Build history of the part. All positions in model axes, mm. A direction names the side the tool comes from. Round coordinates to 2 decimals unless told otherwise and drop trailing zeros. Write each loop counter-clockwise with the first axis right and the second up, starting at its lowest first coordinate (ties: lowest second). Pieces come first, ordered by that corner, then holes. Notation, with made-up numbers: (49.25, 19.5) - (54.25, 19.5) arc R26 cw to (54.25, 35.5) - close; hole circle Ø7 at (51.25, -8). An arc over 180 degrees is marked (long way). Answer as a JSON object with one key per item and string values. Group by question number.
Item 1: Two-plate mould, pull along Y, no slides. Class faces 4 (the flat face through (-1, -11.684, -3)), 5 (the cylindrical face through (4.851, -9.945, -0.888)), 6 (the cylindrical face through (-4.841, -9.117, 0.41)), 7 (the flat face through (-5.207, -10, 0)): +Y half, -Y half, draft (parallel to the pull), parting line (faces both ways), or undercut.
Item 2: Flat gauge pins, fed straight in: pin 1 (1.5 mm diameter, centred on x = 3, z = 0.5, fed in from -Y); pin 2 (5 mm diameter, centred on y = 8.5, z = -4, fed in from -X); pin 3 (1.5 mm diameter, centred on x = -2.5, y = 1.5, fed in from -Z). Where does each tip first touch, or does it go through?
Item 3: Probe line 1 (Y direction, x = -2, z = -4.5); line 2 (Z direction, x = 0, y = 6.5); line 3 (Z direction, x = -2.75, y = 1.25). List the from-to ranges inside material, lowest first. Write a range as from..to.
Item 4: Slice it at B-B, the plane y = 3.5. List the corners of the cut face in (x, z), then the cut area to 3 significant figures.
Item 5: Which spindle directions (+Z, -Z, +X, -X, +Y, -Y) get a long thin tool onto all of the face, cutting with end or side? Do faces 1 (the flat face through (5.207, -10, 0)), 2 (the cylindrical face through (-2.092, 1.002, -5.045)), 3 (the flat face through (-5, 2.032, 0)). Say none if no direction does.
Item 6: Slice it at A-A, the plane y = -6. List the corners of the cut face in (x, z).
from build123d import *

# Parameters (mm, degrees)
SKETCH2_R           = 4.826
BOSS_EXTRUDE1_DEPTH = 15.494
FILLET1_R           = 4.826
SKETCH3_R           = 5.461
BOSS_EXTRUDE2_DEPTH = 2.032
SKETCH4_R           = 4.572
BOSS_EXTRUDE3_DEPTH = 11.684
SKETCH5_R           = 2.921
BOSS_EXTRUDE4_DEPTH = 2.794
BOSS_EXTRUDE4_TAPER = 35
FILLET2_R           = 1.27
FILLET3_R           = 0.508
SKETCH6_R           = 0.889
BOSS_EXTRUDE5_DEPTH = 5.207


with BuildPart() as part:
    # Sketch2 → Boss-Extrude1 (new body)
    with BuildSketch(Plane(origin=(0, 0, 0), x_dir=(1, 0, 0), z_dir=(0, 1, 0))):
        with Locations(Location((0, 0, 0), (0, 0, 270))):  # turned: the seam where the file's is
            Circle(SKETCH2_R)
    extrude(amount=BOSS_EXTRUDE1_DEPTH)

    # Fillet1
    fillet1_edges = [part.edges().sort_by_distance(p)[0] for p in [
        (0, 15.494, -4.826),
    ]]
    fillet(fillet1_edges, radius=FILLET1_R)

    # Sketch3 → Boss-Extrude2 (add)
    with BuildSketch(Plane.XZ):
        with Locations(Location((0, 0, 0), (0, 0, 270))):  # turned: the seam where the file's is
            Circle(SKETCH3_R)
    extrude(amount=-BOSS_EXTRUDE2_DEPTH)

    # Sketch4 → Boss-Extrude3 (add)
    with BuildSketch(Plane.XZ):
        with Locations(Location((0, 0, 0), (0, 0, 90))):  # turned: the seam where the file's is
            Circle(SKETCH4_R)
    extrude(amount=BOSS_EXTRUDE3_DEPTH)

    # Sketch5 → Boss-Extrude4 (add)
    with BuildSketch(Plane.XZ.offset(11.684)):
        Circle(SKETCH5_R)
    extrude(amount=BOSS_EXTRUDE4_DEPTH, taper=BOSS_EXTRUDE4_TAPER)

    # Fillet2
    fillet2_edges = [part.edges().sort_by_distance(p)[0] for p in [
        (-0.964620138, -14.478, 0),
    ]]
    fillet(fillet2_edges, radius=FILLET2_R)

    # Fillet3
    fillet3_edges = [part.edges().sort_by_distance(p)[0] for p in [
        (0, -11.684, -4.572),
    ]]
    fillet(fillet3_edges, radius=FILLET3_R)

    # Sketch6 → Boss-Extrude5 (add, symmetric)
    with BuildSketch(Plane(origin=(0, 0, 0), x_dir=(0, 0, -1), z_dir=(1, 0, 0))):
        with Locations(Location((0, -9.906, 0), (0, 0, 180))):  # turned: the seam where the file's is
            Circle(SKETCH6_R)
    extrude(amount=BOSS_EXTRUDE5_DEPTH, both=True)


solid = part.part
Geometry says:
{
 "1": {"face 4": "-Y half", "face 5": "undercut", "face 6": "undercut", "face 7": "draft"},
 "2": {"pin 1": "stops at y = -12.58", "pin 2": "stops at x = -4.59", "pin 3": "stops at z = -5.17"},
 "3": {"line 1": "y = 0..2.03", "line 2": "z = -4.83..4.83", "line 3": "z = -4.72..4.72"},
 "4": {"outline": "circle Ø9.65 at (0, 0)", "area": "73.2 mm^2"},
 "5": {"face 1": "+Z, -Z, +X, -Y", "face 2": "+Y, -Y", "face 3": "+Y"},
 "6": {"outline": "circle Ø9.14 at (0, 0)"}
}
